The listing builds one solid part. Answer for the finished solid, in the listing's coordinates (mm). Face numbers are marked on the shaded views. A direction names the side the tool comes from. Give positions to 0.01 mm unless a question says otherwise; leave off trailing zeros. Order: outer loops, then holes, each group sorted by start corner. A loop starts at its lowest first (then second) coordinate and runs counter-clockwise, first axis right, second up. Notation, with made-up numbers: (38.5, -34.75) - (93.5, -34.75) arc R29 cw to (93.5, -11.75) - close; hole circle Ø3 at (10, -13). An arc over 180 degrees is marked (long way). Answer in a Markdown table with one row per item. Add a question column.
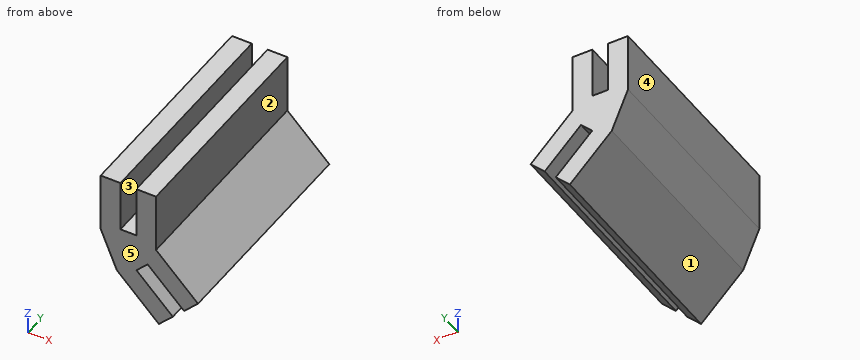
```python
from build123d import *

# Parameters (mm, degrees)
BOSS_EXTRUDE1_DEPTH = 55.374093082
CHAMFER1_START      = -16
CHAMFER1_OUTLINE_W  = 58
CHAMFER1_OUTLINE_H  = 14
CHAMFER1_DEPTH      = 3.065686545


with BuildPart() as part:
    # Sketch2 → Boss-Extrude1 (new body)
    with BuildSketch(Plane(origin=(0, 0, 0), x_dir=(1, 0, 0), z_dir=(0, 1, 0))):
        Polygon((0, 0), (0, -15), (-5, -15), (-5, -2), (-9, -2), (-9, -15), (-14, -15), (-14, 5.798989873), align=None)
    boss_extrude1 = extrude(amount=BOSS_EXTRUDE1_DEPTH)

    # Mirror2: Boss-Extrude1 across plane
    add(boss_extrude1.mirror(Plane(origin=(0, 55.374093082, 0), x_dir=(0.9238795325112891, 0, 0.382683432365084), z_dir=(-0.382683432365084, 0, 0.9238795325112892))))

    # Chamfer1: read off the stored shape, not the designer's step
    # Chamfer1 outline → Chamfer1 (cut)
    with BuildSketch(Plane(origin=(0, 0, 0), x_dir=(0, 1, 0), z_dir=(0.9238795325112892, 0, 0.3826834323650841)).offset(CHAMFER1_START)):
        with Locations((28, 0)):
            Rectangle(CHAMFER1_OUTLINE_W, CHAMFER1_OUTLINE_H)
    extrude(amount=CHAMFER1_DEPTH, mode=Mode.SUBTRACT)


solid = part.part
```
(1) Find section A-A, the plane z = 11.5. Write down the section's boundary in (x, y), plus the area to 3 significant figures.
(2) Each of these flat-tipped pins is pushed along its axis until it touches: P1, Ø1.5, axis at y = 46, z = 10, coming from the +X side; P2, Ø8, axis at x = 6, z = 2.5, coming from the +Y side; P3, Ø2, axis at y = 26, z = -14, coming from the -X side; P4, Ø14.5, axis at y = 18.5, z = 5.5, coming from the +X side. Where does it stop, or does it pass through?
(3) Find section C-C, the plane y = 22. Write down the section's boundary in (x, z), plus the area to 3 significant figures.
(4) For the marked faces 1 and 2, determine the directions among +Z, -Z, +X, -X, +Y, -Y from which every point of the face is accessible in a straight line to the end or side of a thin tool.
(5) Find section D-D, the plane z = 1. Write down the section's boundary in (x, y).
(6) Find section B-B, the plane x = -3. Write down the section's boundary in (y, z), plus the area to 3 significant figures.
(7) The mould has two halves that part along X. Classify the marked faces 3, 4 and 5: +X half, -X half, draft (parallel to the pull), parting line (faces both ways), or undercut.
(8) Straight lines are drawn through the part: line 1 (X direction, y = 18.5, z = 13); line 2 (X direction, y = 49, z = -13); line 3 (Z direction, x = -2.25, y = 16.5). For each, find the intervals that lie inside material, in ascending order.
Answer key:
| question | item | result |
|---|---|---|
| 1 | outline | (-14, 0) - (-9, 0) - (-9, 55.37) - (-14, 55.37) - close; (-5, 0) - (0, 0) - (0, 55.37) - (-5, 55.37) - close |
| 1 | area | 554 mm² |
| 2 | P1 | x = 0 |
| 2 | P2 | through |
| 2 | P3 | x = -6.8 |
| 2 | P4 | x = 1.75 |
| 3 | outline | (-14, 0) - (-9.9, -9.9) - (0.71, -20.51) - (4.24, -16.97) - (-4.95, -7.78) - (-2.12, -4.95) - (7.07, -14.14) - (10.61, -10.61) - (0, 0) - (0, 15) - (-5, 15) - (-5, 2) - (-9, 2) - (-9, 15) - (-14, 15) - close |
| 3 | area | 385 mm² |
| 4 | face 1 | -Z, -X, +Y, -Y |
| 4 | face 2 | +Z, +X, +Y, -Y |
| 5 | outline | (-14, 0) - (0, 0) - (0, 55.37) - (-14, 55.37) - close |
| 6 | outline | (0, -16.8) - (55.37, -16.8) - (55.37, -9.73) - (0, -9.73) - close; (0, -5.83) - (55.37, -5.83) - (55.37, 15) - (0, 15) - close |
| 6 | area | 1,540 mm² |
| 7 | face 3 | undercut |
| 7 | face 4 | -X half |
| 7 | face 5 | draft |
| 8 | line 1 | -14 to -9, -5 to 0 |
| 8 | line 2 | -6.8 to 0.27, 5.93 to 8.21 |
| 8 | line 3 | -17.55 to -10.48, -5.08 to 15 |
